Could you check a few things on this model? Use its own coordinates, in mm. Coordinates: 2 decimals unless noted, no trailing zeros. Loops run counter-clockwise (first coordinate to the right, second up) from the corner with the lowest first, then second, coordinate; pieces in that order, holes last. Notation, with made-up numbers: (83.25, 43) - (121.25, 43) arc R8 ccw to (121.25, 57) - close; hole circle Ø7 at (61, -4.5). An arc over 180 degrees is marked (long way). Use CSV: the item, a comma, the result in double quotes.
from build123d import *

# Parameters (mm, degrees)
SKETCH_1_W           = 38
SKETCH_1_H           = 38
SKETCH_1_R           = 1.5
EXTRUDE_1_DEPTH      = 1.5
SKETCH_2_W           = 5
SKETCH_2_H           = 26.5
SKETCH_2_W_2         = 30.5
SKETCH_2_H_2         = 3
EXTRUDE_2_DEPTH      = 1.5
EXTRUDE_3_DEPTH      = 3
EXTRUDE_3_DEPTH_BACK = 4.5
SKETCH_3_W           = 25
SKETCH_3_H           = 25


with BuildPart() as part:
    # 草图1 → 凸台-拉伸1 (new body)
    with BuildSketch(Plane(origin=(0, 0, 0), x_dir=(1, 0, 0), z_dir=(0, 1, 0))):
        Rectangle(SKETCH_1_W, SKETCH_1_H)
        with Locations(Location((-15.25, 15.25, 0), (0, 0, 270))):
            Circle(SKETCH_1_R, mode=Mode.SUBTRACT)
        with Locations(Location((15.25, 15.25, 0), (0, 0, 270))):
            Circle(SKETCH_1_R, mode=Mode.SUBTRACT)
        with Locations(Location((15.25, -15.25, 0), (0, 0, 270))):
            Circle(SKETCH_1_R, mode=Mode.SUBTRACT)
        with Locations(Location((-15.25, -15.25, 0), (0, 0, 270))):
            Circle(SKETCH_1_R, mode=Mode.SUBTRACT)
    extrude(amount=EXTRUDE_1_DEPTH)

    # 草图2 → 凸台-拉伸2 (add)
    with BuildSketch(Plane.XZ):
        with Locations((-21.5, 0)):
            Rectangle(SKETCH_2_W, SKETCH_2_H)
        with Locations((0, -20.5)):
            Rectangle(SKETCH_2_W_2, SKETCH_2_H_2)
        with Locations((0, 20.5)):
            Rectangle(SKETCH_2_W_2, SKETCH_2_H_2)
    extrude(amount=-EXTRUDE_2_DEPTH)

    # 草图3 → 凸台-拉伸3 (add, two sides: drawn at the far end of the back side and taken through both)
    with BuildSketch(Plane(origin=(0, 1.5, 0), x_dir=(1, 0, 0), z_dir=(0, 1, 0)).offset(-EXTRUDE_3_DEPTH_BACK)):
        Rectangle(SKETCH_3_W, SKETCH_3_H)
    extrude(amount=EXTRUDE_3_DEPTH + EXTRUDE_3_DEPTH_BACK)


solid = part.part
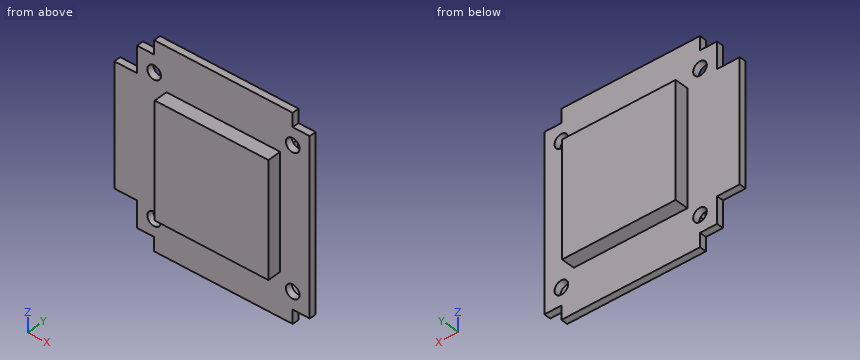
(1) Suppose I cut it at A-A (z = -15.25). Write out the boundary of the cut face in (x, y), plus the area to 3 significant figures.
Computed:
outline,"(-19, 0) - (-16.75, 0) - (-16.75, 1.5) - (-19, 1.5) - close; (-13.75, 0) - (13.75, 0) - (13.75, 1.5) - (-13.75, 1.5) - close; (16.75, 0) - (19, 0) - (19, 1.5) - (16.75, 1.5) - close"
area,"48.0 mm²"
(2) Suppose I cut it at C-C (z = -1.5). Write out the boundary of the cut face in (x, y), plus the area to 4 significant figures.
Computed:
outline,"(-24, 0) - (-12.5, 0) - (-12.5, -3) - (12.5, -3) - (12.5, 0) - (19, 0) - (19, 1.5) - (12.5, 1.5) - (12.5, 4.5) - (-12.5, 4.5) - (-12.5, 1.5) - (-24, 1.5) - close"
area,"214.5 mm²"
(3) Will these pins go through, and if not, where does the flat tip stop? pin 1 (1 mm diameter, centred on y = 3, z = 15, fed in from +X); pin 2 (1.2 mm diameter, centred on y = 0.5, z = -21, fed in from +X); pin 3 (1.6 mm diameter, centred on x = 16.5, y = 0.5, fed in from +Z); pin 4 (3 mm diameter, centred on x = -8.5, z = 15.5, fed in from +Y).
Computed:
pin 1,"passes through"
pin 2,"stops at x = 15.25"
pin 3,"stops at z = 19"
pin 4,"stops at y = 1.5"
(4) Suppose I cut it at D-D (y = 2). Write out the boundary of the cut face in (x, z), plus the area to 3 significant figures.
Computed:
outline,"(-12.5, -12.5) - (12.5, -12.5) - (12.5, 12.5) - (-12.5, 12.5) - close"
area,"625 mm²"
(5) Suppose I cut it at B-B (x = 4.5). Write out the boundary of the cut face in (y, z).
Computed:
outline,"(-3, -12.5) - (0, -12.5) - (0, -22) - (1.5, -22) - (1.5, -12.5) - (4.5, -12.5) - (4.5, 12.5) - (1.5, 12.5) - (1.5, 22) - (0, 22) - (0, 12.5) - (-3, 12.5) - close"
(6) Please list where these lines run through material, in increasing order: line 1 (X direction, y = 0.7, z = -15.25); line 2 (Z direction, x = -14, y = 0.25); line 3 (Y direction, x = 13, z = 14.5).
Computed:
line 1,"x = -19 to -16.75, -13.75 to 13.75, 16.75 to 19"
line 2,"z = -22 to -16.08, -14.42 to 14.42, 16.08 to 22"
line 3,"y = 0 to 1.5"
